The listing builds one solid part. Answer for the finished solid, in the listing's coordinates (mm). Coordinates: 2 decimals unless noted, no trailing zeros. Order: outer loops, then holes, each group sorted by start corner. A loop starts at its lowest first (then second) coordinate and runs counter-clockwise, first axis right, second up. Notation, with made-up numbers: (-0.5, 85) -> (13.5, 85) arc R27 cw to (13.5, 107) -> close; hole circle Ø4 at (74.5, 28.25). An arc over 180 degrees is marked (long way). Put each result on its own line as item: value. Start each with the question number.
Autodesk Inventor part; units mm, degrees
ref_plane "YZ Plane" through (0, 0, 0) normal (1, 0, 0) x (0, 1, 0)
ref_plane "XZ Plane" through (0, 0, 0) normal (0, 1, 0) x (-1, 0, 0)
ref_plane "XY Plane" through (0, 0, 0) normal (0, 0, 1) x (1, 0, 0)
sketch "Sketch1" plane through (0, 0, 0) normal (0, 1, 0) x (-1, 0, 0)
  line L0 (99, 89) -> (-99, 89)
  line L1 (-99, 89) -> (-99, -89)
  line L2 (-99, -89) -> (99, -89)
  line L3 (99, -89) -> (99, 89)
  line L4 (99, 89) -> (-99, -89) construction
  line L5 (-99, 89) -> (99, -89) construction
  line L6 (-99, 89) -> (-85, 89)
  line L7 (-85, 89) -> (-85, -89)
  line L8 (-85, -89) -> (-99, -89)
  line L9 (-99, -89) -> (-99, 89)
  line L10 (99, 89) -> (97, 89)
  line L11 (97, 89) -> (97, -89)
  line L12 (97, -89) -> (99, -89)
  line L13 (99, -89) -> (99, 89)
  line L14 (97, 33) -> (97, 35)
  line L15 (97, -33) -> (97, -35)
  line L16 (97, 32.8) -> (97, 35)
  line L17 (97, -32.8) -> (97, -35)
  line L18 (97, 89) -> (47, 89)
  line L19 (47, 89) -> (47, 34)
  line L20 (47, 34) -> (97, 34)
  line L21 (97, 34) -> (97, 89)
  line L22 (97, -89) -> (47, -89)
  line L23 (47, -89) -> (47, -34)
  line L24 (47, -34) -> (97, -34)
  line L25 (97, -34) -> (97, -89)
  line L26 (66.5, 33) -> (77.5, 33)
  line L27 (77.5, -33) -> (66.5, -33)
  point P0 (0, 0)
  point P1 (47, 89)
  point P2 (47, -89)
  point P3 (97, 34)
  dimension "d0" = 198
  dimension "d1" = 178
  dimension "d2" = 14
  dimension "d3" = 2
  dimension "d16" = 50
  dimension "d17" = 55
  dimension "d18" = 50
  dimension "d19" = 55
  dimension "d20" = 1
  dimension "d21" = 1
extrude "Extrusion1" add sketch "Sketch1" along normal blind 3.5 contours L19 L20 L11 L24 L23 L2 L7 L0
properties part number "base" material "Nylon 6/6"
(1) Find the intervals of material crossed by L1, parallel to X at y = 2.6, z = 66, in increasing order.
(2) The part is cut by section B-B on x = -58. Determine the outline of the cut face in (y, z), plus the area to 3 significant figures.
(3) Each of these flat-tipped pins is pushed along its axis until it touches: P1, Ø1.8, axis at x = -76.5, y = 1, coming from the -Z side; P2, Ø1.8, axis at y = 1, z = 65, coming from the -X side. Where does it stop, or does it pass through?
(4) The part is cut by section C-C on z = 48.5. Determine the outline of the cut face in (x, y).
(5) The part is cut by section A-A on y = 2.45. Determine the outline of the cut face in (x, z).
Worked out:
1. L1: -47 to 85
2. outline: (0, -34) -> (3.5, -34) -> (3.5, 34) -> (0, 34) -> close
2. area: 238 mm2
3. P1: z = -34
3. P2: x = -47
4. outline: (-47, 0) -> (85, 0) -> (85, 3.5) -> (-47, 3.5) -> close
5. outline: (-97, -34) -> (-47, -34) -> (-47, -89) -> (85, -89) -> (85, 89) -> (-47, 89) -> (-47, 34) -> (-97, 34) -> close
